```python
from build123d import *

# Parameters (mm, degrees)
SKETCH1_W               = 25.4
SKETCH1_H               = 76.2
SKETCH1_W_2             = 19.05
SKETCH1_H_2             = 69.85
BOSS_EXTRUDE3_DEPTH     = 254
SKETCH6_R               = 3.175
CUT_EXTRUDE1_DEPTH      = 806.45
CUT_EXTRUDE2_DEPTH      = 266.487720997
CUT_EXTRUDE2_DEPTH_BACK = 266.487720997
SKETCH7_R               = 3.175
CUT_EXTRUDE4_DEPTH      = 266.487720997
CUT_EXTRUDE4_DEPTH_BACK = 266.487720997
SKETCH8_R               = 3.175
CUT_EXTRUDE6_DEPTH      = 259.094498198
CUT_EXTRUDE6_DEPTH_BACK = 259.094498198
SKETCH11_R              = 3.175


with BuildPart() as part:
    # Sketch1 → Boss-Extrude3 (new body)
    with BuildSketch(Plane.XY):
        Rectangle(SKETCH1_W, SKETCH1_H)
        Rectangle(SKETCH1_W_2, SKETCH1_H_2, mode=Mode.SUBTRACT)
    extrude(amount=BOSS_EXTRUDE3_DEPTH)

    # Sketch6 → Cut-Extrude1 (cut)
    with BuildSketch(Plane(origin=(0, -38.1, 0), x_dir=(-1, 0, 0), z_dir=(0, -1, 0))):
        with Locations(Location((0, -12.7, 0), (0, 0, 180))):
            Circle(SKETCH6_R)
        with Locations(Location((0, -38.1, 0), (0, 0, 180))):
            Circle(SKETCH6_R)
        with Locations(Location((0, -241.3, 0), (0, 0, 180))):
            Circle(SKETCH6_R)
        with Locations(Location((0, -215.9, 0), (0, 0, 180))):
            Circle(SKETCH6_R)
    extrude(amount=-CUT_EXTRUDE1_DEPTH, mode=Mode.SUBTRACT)

    # Sketch7 → Cut-Extrude2 (cut, two sides: drawn at the far end of the back side and taken through both)
    with BuildSketch(Plane(origin=(0, -38.1, 0), x_dir=(-1, 0, 0), z_dir=(0, -1, 0)).offset(-CUT_EXTRUDE2_DEPTH_BACK)):
        with Locations(Location((0, -88.9, 0), (0, 0, 180))):
            Circle(SKETCH7_R)
        with Locations(Location((0, -114.3, 0), (0, 0, 180))):
            Circle(SKETCH7_R)
        with Locations(Location((0, -165.1, 0), (0, 0, 180))):
            Circle(SKETCH7_R)
        with Locations(Location((0, -139.7, 0), (0, 0, 180))):
            Circle(SKETCH7_R)
    extrude(amount=CUT_EXTRUDE2_DEPTH + CUT_EXTRUDE2_DEPTH_BACK, mode=Mode.SUBTRACT)

    # Sketch8 → Cut-Extrude4 (cut, two sides: drawn at the far end of the back side and taken through both)
    with BuildSketch(Plane(origin=(0, -38.1, 0), x_dir=(-1, 0, 0), z_dir=(0, -1, 0)).offset(-CUT_EXTRUDE4_DEPTH_BACK)):
        with Locations(Location((0, -190.5, 0), (0, 0, 180))):
            Circle(SKETCH8_R)
        with Locations(Location((0, -215.9, 0), (0, 0, 180))):
            Circle(SKETCH8_R)
        with Locations(Location((0, -63.5, 0), (0, 0, 180))):
            Circle(SKETCH8_R)
        with Locations(Location((0, -38.1, 0), (0, 0, 180))):
            Circle(SKETCH8_R)
    extrude(amount=CUT_EXTRUDE4_DEPTH + CUT_EXTRUDE4_DEPTH_BACK, mode=Mode.SUBTRACT)

    # Sketch11 → Cut-Extrude6 (cut, two sides: drawn at the far end of the back side and taken through both)
    with BuildSketch(Plane(origin=(12.7, 0, 0), x_dir=(0, 0, -1), z_dir=(1, 0, 0)).offset(-CUT_EXTRUDE6_DEPTH_BACK)):
        with Locations((-241.3, -25.4)):
            Circle(SKETCH11_R)
        with Locations((-215.9, -25.4)):
            Circle(SKETCH11_R)
        with Locations((-215.9, 25.4)):
            Circle(SKETCH11_R)
        with Locations((-241.3, 25.4)):
            Circle(SKETCH11_R)
    extrude(amount=CUT_EXTRUDE6_DEPTH + CUT_EXTRUDE6_DEPTH_BACK, mode=Mode.SUBTRACT)


solid = part.part
```
Part model, mm, in its own coordinate system. Round coordinates to 2 decimals unless told otherwise and drop trailing zeros. Write each loop counter-clockwise with the first axis right and the second up, starting at its lowest first coordinate (ties: lowest second). Pieces come first, ordered by that corner, then holes. Notation, with made-up numbers: (1, 55) -> (33, 55) arc R7 cw to (33, 64) -> close; hole circle Ø11 at (9.25, -22.75). An arc over 180 degrees is marked (long way). Return JSON: item names as keys, results as strings. Group by question number.
Q1. Pin check, flat tip, straight feed: pin 1 (4 mm diameter, centred on x = 0, z = 12.7, fed in from +Y). Stop position of the tip, or through.
Q2. Saw through at C-C on z = 12.7. Write the cut outline in (x, y) (3 decimals).
Q3. Saw through at B-B on y = 18.5. Write the cut outline in (x, z) (3 decimals), plus the area to 3 significant figures.
Q4. Saw through at D-D on z = 97. Write the cut outline in (x, y) (3 decimals), plus the area to 3 significant figures.
Q5. Saw through at A-A on z = 215.9. State how many separate pieces and enclosed holes the cut face has, plus the area to 3 significant figures.
Q6. Probe L1, parallel to Y at x = 10.2, z = 241.3 (3 decimals); L2, parallel to X at y = -2.5, z = 188 (3 decimals); L3, parallel to Y at x = 8, z = 94 (3 decimals). List the from-to ranges inside material, lowest first. Write a range as [from, to].
Q7. Mould opens along X. For faces 1 (the flat face through (-10, 3, 0)), 2 (the cylindrical face through (-0.69, 36.49, 35)), 3 (the cylindrical face through (-0.69, 36.53, 85.8)) say: pulls with the +X half, pulls with the -X half, needs draft (parallel to the pull), parting line crosses it, or undercut.
Answer:
{
 "1": {"pin 1": "through"},
 "2": {"outline": "(-12.7, -38.1) -> (-3.175, -38.1) -> (-3.175, -34.925) -> (-9.525, -34.925) -> (-9.525, 34.925) -> (-3.175, 34.925) -> (-3.175, 38.1) -> (-12.7, 38.1) -> close; (3.175, -38.1) -> (12.7, -38.1) -> (12.7, 38.1) -> (3.175, 38.1) -> (3.175, 34.925) -> (9.525, 34.925) -> (9.525, -34.925) -> (3.175, -34.925) -> close"},
 "3": {"outline": "(-12.7, 0) -> (-9.525, 0) -> (-9.525, 254) -> (-12.7, 254) -> close; (9.525, 0) -> (12.7, 0) -> (12.7, 254) -> (9.525, 254) -> close", "area": "1,610 mm2"},
 "4": {"outline": "(-12.7, -38.1) -> (12.7, -38.1) -> (12.7, 38.1) -> (-12.7, 38.1) -> close; hole (-9.525, -34.925) -> (9.525, -34.925) -> (9.525, 34.925) -> (-9.525, 34.925) -> close", "area": "605 mm2"},
 "5": {"separate pieces": "6", "enclosed holes": "0", "area": "484 mm2"},
 "6": {"L1": "[-38.1, -28.575], [-22.225, 22.225], [28.575, 38.1]", "L2": "[-12.7, -9.525], [9.525, 12.7]", "L3": "[-38.1, -34.925], [34.925, 38.1]"},
 "7": {"face 1": "needs draft", "face 2": "undercut", "face 3": "undercut"}
}
